```python
from build123d import *

# Parameters (mm, degrees)
SKETCH1_W            = 28
SKETCH1_H            = 32
BOSS_EXTRUDE1_DEPTH  = 5
M3_CLEARANCE_HOLE1_D = 3.4
BOSS_EXTRUDE2_DEPTH  = 7
FILLET1_R            = 10
FILLET2_R            = 5
FILLET3_R            = 5
M3_CLEARANCE_HOLE2_D = 3.4
CHAMFER1_SIZE        = 25
CHAMFER1_SIZE2       = 9.099255857


with BuildPart() as part:
    # Sketch1 → Boss-Extrude1 (new body)
    with BuildSketch(Plane(origin=(0, 0, 0), x_dir=(1, 0, 0), z_dir=(0, 1, 0))):
        Rectangle(SKETCH1_W, SKETCH1_H)
    extrude(amount=BOSS_EXTRUDE1_DEPTH)

    # M3 Clearance Hole1 (through all)
    with Locations(Plane(origin=(0, 5, 0), x_dir=(1, 0, 0), z_dir=(0, 1, 0))):
        with Locations((-6, 8), (6, 8), (6, 0), (-6, 0)):
            Hole(M3_CLEARANCE_HOLE1_D / 2)

    # Sketch5 → Boss-Extrude2 (add)
    with BuildSketch(Plane.XY.offset(16)):
        Polygon((-14, 0), (-62, 0), (-62, 43), (-49, 43), (-49, 24), (-27, 24), (-27, 43), (-14, 43), align=None)
    extrude(amount=-BOSS_EXTRUDE2_DEPTH)

    # Fillet1
    fillet1_edges = [part.edges().sort_by_distance(p)[0] for p in [
        (-49, 24, 12.5),
        (-27, 24, 12.5),
    ]]
    fillet(fillet1_edges, radius=FILLET1_R)

    # Fillet2
    fillet2_edges = [part.edges().sort_by_distance(p)[0] for p in [
        (-14, 5, 12.5),
    ]]
    fillet(fillet2_edges, radius=FILLET2_R)

    # Fillet3
    fillet3_edges = [part.edges().sort_by_distance(p)[0] for p in [
        (-14, 2.5, 9),
    ]]
    fillet(fillet3_edges, radius=FILLET3_R)

    # M3 Clearance Hole2 (through all)
    with Locations(Plane.XY.offset(16)):
        with Locations((-53, 35), (-23, 35), (-38, 20)):
            Hole(M3_CLEARANCE_HOLE2_D / 2)

    # Chamfer1
    chamfer1_edges = [part.edges().sort_by_distance(p)[0] for p in [
        (-62, 0, 12.5),
    ]]
    chamfer1_side = [part.faces().sort_by_distance(p)[0] for p in [
        (-10.698240226, 0, 3.653109537),
    ]]
    chamfer(chamfer1_edges, length=CHAMFER1_SIZE, length2=CHAMFER1_SIZE2, reference=chamfer1_side[0])


solid = part.part
```
Geometry: final body of the model. Coordinates: model frame, mm. A direction names the side the tool comes from. Give positions to 0.01 mm unless a question says otherwise; leave off trailing zeros. Order: outer loops, then holes, each group sorted by start corner. A loop starts at its lowest first (then second) coordinate and runs counter-clockwise, first axis right, second up. Notation, with made-up numbers: M 64,11.25 L 96,11.25 A16 ccw 96,24.25 Z; hole C -31.5,36.5 d1. An arc over 180 degrees is marked long. Answer as CSV lines item,"result". Start each with the question number.
1) Line query: line 1 (X direction, y = 1, z = -8); line 2 (Z direction, x = -6, y = 2.4); line 3 (Z direction, x = 7, y = 3). Output: solid intervals per line, ascending. Write a range as from..to.
2) Cut plane B-B (y = 26). Output: boundary loops of the cut face in (x, z), then the cut area to 3 significant figures.
3) Mould query, pull axis X, two halves, no side actions, for faces 1 (the flat face through (-49, 39, 13)), 2 (the flat face through (14, 2, 0)), 3 (the flat face through (-21, 43, 13)), 4 (the cylindrical face through (6.37, 2.46, 1.66)). Classes: +X half, -X half, draft (parallel to the pull), parting line (faces both ways), or undercut.
4) Cut plane D-D (x = -23). Output: boundary loops of the cut face in (y, z).
5) Set-up query: faces 5 (the flat face through (1, 5, 0)), 6 (the cylindrical face through (-4.65, 2.46, 1.03)). Return all of +Z, -Z, +X, -X, +Y, -Y with unobstructed straight access to the full face (end or side cutting, diameter ignored); none if empty.
6) Cut plane C-C (y = 35). Output: boundary loops of the cut face in (x, z), then the cut area to 3 significant figures.
7) Cut plane A-A (x = 6). Output: boundary loops of the cut face in (y, z).
8) First-contact query: P1, Ø16, axis at x = -6.5, z = -3.5, coming from the +Y side; P2, Ø5.5, axis at x = -38, y = 20, coming from the -Z side; P3, Ø2, axis at x = -38, z = 12.5, coming from the +Y side; P4, Ø4, axis at x = -53, y = 35, coming from the +Z side. Flat tips, straight axial feed; report the tip coordinate or a pass-through.
Findings below:
1,line 1,"x = -14..-7.7, -4.3..4.3, 7.7..14"
1,line 2,"z = -16..-9.7, -6.3..-1.7, 1.7..16"
1,line 3,"z = -16..-9.37, -6.63..-1.37, 1.37..16"
2,outline,"M -62,9 L -45,9 L -45,16 L -62,16 Z; M -31,9 L -14,9 L -14,16 L -31,16 Z"
2,area,"238 mm²"
3,face 1,"undercut"
3,face 2,"+X half"
3,face 3,"draft"
3,face 4,"undercut"
4,outline,"M 0,9 L 33.3,9 L 33.3,16 L 0,16 Z; M 36.7,9 L 43,9 L 43,16 L 36.7,16 Z"
5,face 5,"-Z, +X, +Y"
5,face 6,"+Y, -Y"
6,outline,"M -62,9 L -54.7,9 L -54.7,16 L -62,16 Z; M -51.3,9 L -49,9 L -49,16 L -51.3,16 Z; M -27,9 L -24.7,9 L -24.7,16 L -27,16 Z; M -21.3,9 L -14,9 L -14,16 L -21.3,16 Z"
6,area,"134 mm²"
7,outline,"M 0,-16 L 5,-16 L 5,-9.7 L 0,-9.7 Z; M 0,-6.3 L 5,-6.3 L 5,-1.7 L 0,-1.7 Z; M 0,1.7 L 5,1.7 L 5,16 L 0,16 Z"
8,P1,"stops at y = 5"
8,P2,"stops at z = 9"
8,P3,"stops at y = 24"
8,P4,"stops at z = 16"
